from build123d import *

# Parameters (mm, degrees)
SKETCH1_R           = 1.7
BOSS_EXTRUDE1_DEPTH = 5
SKETCH2_R           = 1.7
BOSS_EXTRUDE2_DEPTH = 5
SKETCH3_R           = 10
SKETCH3_R_2         = 5
BOSS_EXTRUDE3_DEPTH = 5
SKETCH4_R           = 5
CUT_EXTRUDE1_DEPTH  = 5


with BuildPart() as part:
    # Sketch1 → Boss-Extrude1 (new body)
    with BuildSketch(Plane(origin=(0, 0, 0), x_dir=(1, 0, 0), z_dir=(0, 1, 0))):
        with BuildLine():
            Line((-5, 0), (-5, 45))
            ThreePointArc((-5, 45), (0, 50), (5, 45))
            Line((5, 45), (5, 0))
            ThreePointArc((5, 0), (0, -5), (-5, 0))
        make_face()
        with Locations(Location((0, 0, 0), (0, 0, 270))):
            Circle(SKETCH1_R, mode=Mode.SUBTRACT)
        with Locations(Location((0, 45, 0), (0, 0, 270))):
            Circle(SKETCH1_R, mode=Mode.SUBTRACT)
    extrude(amount=BOSS_EXTRUDE1_DEPTH)

    # Sketch2 → Boss-Extrude2 (add)
    with BuildSketch(Plane.XZ):
        with BuildLine():
            Line((0, -40), (45.5, -40))
            ThreePointArc((45.5, -40), (50.5, -45), (45.5, -50))
            Line((45.5, -50), (0, -50))
            ThreePointArc((0, -50), (-5, -45), (0, -40))
        make_face()
        with Locations(Location((45.5, -45, 0), (0, 0, 270))):
            Circle(SKETCH2_R, mode=Mode.SUBTRACT)
        with Locations(Location((0, -45, 0), (0, 0, 90))):
            Circle(SKETCH2_R, mode=Mode.SUBTRACT)
    extrude(amount=-BOSS_EXTRUDE2_DEPTH)

    # Sketch3 → Boss-Extrude3 (add)
    with BuildSketch(Plane.XZ):
        with Locations((45.5, -45)):
            Circle(SKETCH3_R)
        with Locations((45.5, -45)):
            Circle(SKETCH3_R_2, mode=Mode.SUBTRACT)
    extrude(amount=-BOSS_EXTRUDE3_DEPTH)

    # Sketch4 → Cut-Extrude1 (cut)
    with BuildSketch(Plane.XZ):
        with Locations(Location((45.5, -45, 0), (0, 0, 270))):
            Circle(SKETCH4_R)
    extrude(amount=-CUT_EXTRUDE1_DEPTH, mode=Mode.SUBTRACT)


solid = part.part
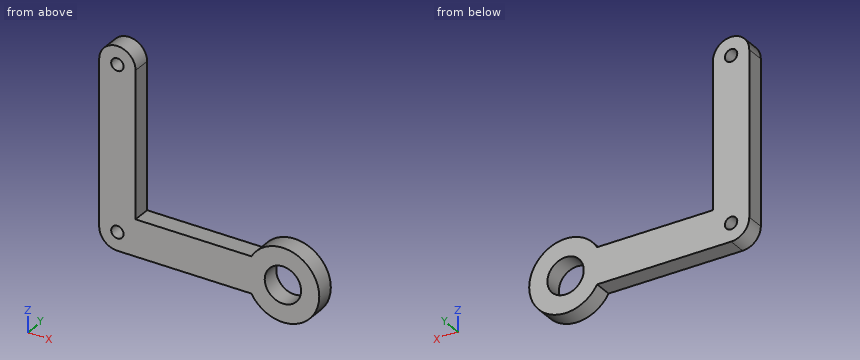
Here's how the part is built. I have some questions about the finished solid (model axes, mm). Coordinates: 2 decimals unless noted, no trailing zeros. Order: outer loops, then holes, each group sorted by start corner. A loop starts at its lowest first (then second) coordinate and runs counter-clockwise, first axis right, second up. Notation, with made-up numbers: M 57,-6 L 105,-6 A26 ccw 105,20 Z; hole C 25.25,79 d3. An arc over 180 degrees is marked long. Answer as CSV lines item,"result". Start each with the question number.
1. For pin 1 (2.5 mm diameter, centred on x = 20, y = 3.5, fed in from -Z), with a flat end and sliding along its axis, tell me the tip position at first contact or that it passes through.
2. I want a section at A-A, the plane x = 45.5. Write out the boundary of the cut face in (y, z).
3. I need wall thicknesses on line 1 (X direction, y = 1.9, z = -45); line 2 (Z direction, x = 25, y = 2.9); line 3 (Z direction, x = 43.5, y = 1.75). Which ranges of each line are inside material? Lowest first, please. Write a range as [from, to].
4. I want a section at C-C, the plane x = 20.5. Write out the boundary of the cut face in (y, z).
5. I want a section at B-B, the plane y = 1.6. Write out the boundary of the cut face in (x, z).
6. I want a section at D-D, the plane z = -25. Write out the boundary of the cut face in (x, y), and give its area (3 significant figures).
Recorded:
1,pin 1,"stops at z = -50"
2,outline,"M 0,-55 L 5,-55 L 5,-50 L 0,-50 Z; M 0,-40 L 5,-40 L 5,-35 L 0,-35 Z"
3,line 1,"x = [-5, -1.7], [1.7, 40.5], [50.5, 55.5]"
3,line 2,"z = [-50, -40]"
3,line 3,"z = [-54.8, -49.58], [-40.42, -35.2]"
4,outline,"M 0,-50 L 5,-50 L 5,-40 L 0,-40 Z"
5,outline,"M -5,-45 A5 ccw 0,-50 L 36.84,-50 A10 ccw long 36.84,-40 L 5,-40 L 5,0 A5 ccw -5,0 Z; hole C 0,-45 d3.4; hole C 0,0 d3.4; hole C 45.5,-45 d10"
6,outline,"M -5,0 L 5,0 L 5,5 L -5,5 Z"
6,area,"50.0 mm2"
